Part model, mm, in its own coordinate system. Round coordinates to 2 decimals unless told otherwise and drop trailing zeros. Loops run counter-clockwise (first coordinate to the right, second up) from the corner with the lowest first, then second, coordinate; pieces in that order, holes last.
(1) Cut at C-C on x = -19. List the corners of the cut face in (y, z), then the cut area to 3 significant figures.
(2) Cut at B-B on y = 58. List the corners of the cut face in (x, z), then the cut area to 3 significant figures.
(3) Probe probe 1 along X at (y, z) = (20, 1.35); probe 2 along Y at (x, z) = (128, 5.75). List the from-to ranges inside material, lowest first.
(4) Flat gauge pins, fed straight in: pin 1 (3 mm diameter, centred on y = 82, z = 2, fed in from +X); pin 2 (0.8 mm diameter, centred on y = 0, z = 5.5, fed in from -X); pin 3 (1.8 mm diameter, centred on x = -70.5, z = 3, fed in from -Y). Where does each tip first touch, or does it go through?
(5) Cut at A-A on x = 87. List the corners of the cut face in (y, z), then the cut area to 3 significant figures.
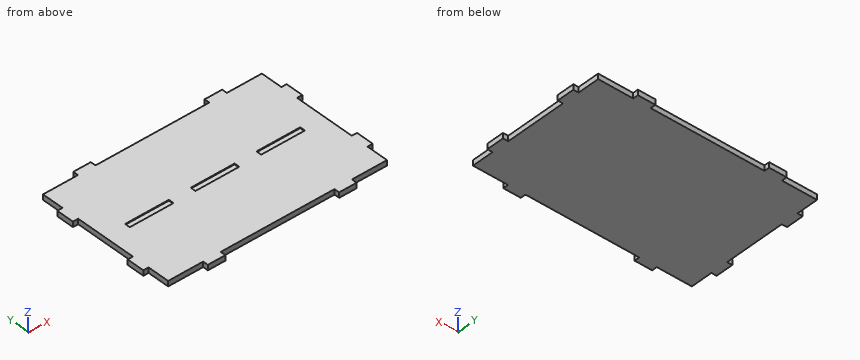
Solid Edge part; units mm, degrees
sketch "Sketch1" plane through (0, 0, 0) normal (0, 0, 1) x (1, 0, 0)
  line L0 (-40, -80) -> (90, -80)
  line L1 (90, -80) -> (90, -86)
  line L2 (90, -86) -> (110, -86)
  line L3 (110, -86) -> (110, -80)
  line L4 (110, -80) -> (150, -80)
  line L5 (150, -80) -> (150, -55)
  line L6 (150, -55) -> (156, -55)
  line L7 (156, -55) -> (156, -35)
  line L8 (156, -35) -> (150, -35)
  line L9 (150, -35) -> (150, 35)
  line L10 (150, 35) -> (156, 35)
  line L11 (156, 35) -> (156, 55)
  line L12 (156, 55) -> (150, 55)
  line L13 (150, 55) -> (150, 80)
  line L14 (150, 80) -> (110, 80)
  line L15 (110, 80) -> (110, 86)
  line L16 (110, 86) -> (90, 86)
  line L17 (90, 86) -> (90, 80)
  line L18 (90, 80) -> (-40, 80)
  line L19 (-40, 80) -> (-40, 86)
  line L20 (-40, 86) -> (-60, 86)
  line L21 (-60, 86) -> (-60, 80)
  line L22 (-60, 80) -> (-100, 80)
  line L23 (-100, 80) -> (-100, 55)
  line L24 (-100, 55) -> (-106, 55)
  line L25 (-106, 55) -> (-106, 35)
  line L26 (-106, 35) -> (-100, 35)
  line L27 (-100, 35) -> (-100, -35)
  line L28 (-100, -35) -> (-106, -35)
  line L29 (-106, -35) -> (-106, -55)
  line L30 (-106, -55) -> (-100, -55)
  line L31 (-100, -55) -> (-100, -80)
  line L32 (-100, -80) -> (-60, -80)
  line L33 (-60, -80) -> (-60, -86)
  line L34 (-60, -86) -> (-40, -86)
  line L35 (-40, -86) -> (-40, -80)
  dimension "D1" = 90
  dimension "D2" = 156
  dimension "D3" = 156
  dimension "D4" = 60
  dimension "D5" = 106
  dimension "D6" = 106
  dimension "D7" = 40
  dimension "D8" = 110
  dimension "D9" = 110
  dimension "D10" = 150
  dimension "D11" = 150
  dimension "D12" = 156
  dimension "D13" = 150
  dimension "D14" = 156
  dimension "D15" = 100
extrude "Protrusion1" add sketch "Sketch1" along normal blind 6
sketch "Sketch2" plane through (25, 0, 6) normal (0, 0, 1) x (1, 0, 0)
  line L0 (-100, -3) -> (-50, -3)
  line L1 (-50, -3) -> (-50, 3)
  line L2 (-50, 3) -> (-100, 3)
  line L3 (-100, 3) -> (-100, -3)
  line L4 (50, -3) -> (100, -3)
  line L5 (100, -3) -> (100, 3)
  line L6 (100, 3) -> (50, 3)
  line L7 (50, 3) -> (50, -3)
  line L8 (-25, -3) -> (25, -3)
  line L9 (25, -3) -> (25, 3)
  line L10 (25, 3) -> (-25, 3)
  line L11 (-25, 3) -> (-25, -3)
  dimension "D1" = 50
  dimension "D2" = 50
  dimension "D3" = 100
  dimension "D4" = 100
  dimension "D5" = 50
extrude "ExtrudedCutout_1" cut sketch "Sketch2" against normal blind 1
Final values:
1. outline: (-80, 0) - (80, 0) - (80, 6) - (-80, 6) - close
1. area: 960 mm2
2. outline: (-100, 0) - (150, 0) - (150, 6) - (-100, 6) - close
2. area: 1,500 mm2
3. probe 1: x = -100 to 150
3. probe 2: y = -80 to 80
4. pin 1: stops at x = 110
4. pin 2: stops at x = -100
4. pin 3: stops at y = -80
5. outline: (-80, 0) - (80, 0) - (80, 6) - (3, 6) - (3, 5) - (-3, 5) - (-3, 6) - (-80, 6) - close
5. area: 954 mm2
